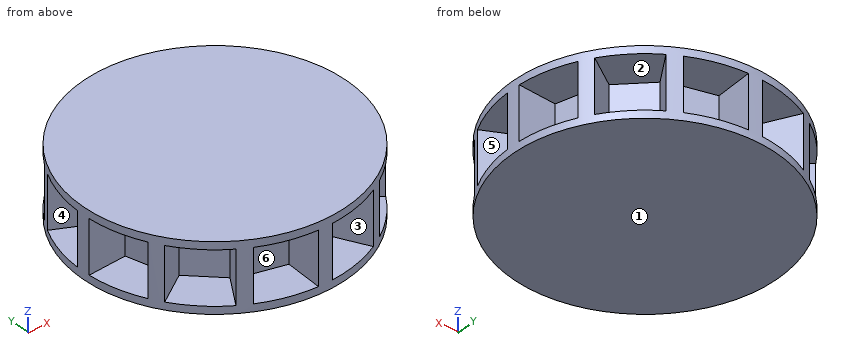
```python
from build123d import *

# Parameters (mm, degrees)
F0_R     = 35
F1_DEPTH = 18
F3_DEPTH = 16
F4_R     = 35
F5_DEPTH = 2


with BuildPart() as f1:
    # F0 (on Top) → F1 (new body)
    with BuildSketch(Plane.XY):
        Circle(F0_R)
    extrude(amount=F1_DEPTH)

    # F2 (on face) → F3 (cut)
    with BuildSketch(Plane(origin=(0, 0, 0), x_dir=(1, 0, 0), z_dir=(0, 0, -1))):
        with BuildLine():
            Line((11.3497624935, 22.2751631047), (15.8896674909, 31.1852283466))
            ThreePointArc((15.8896674909, 31.1852283466), (9.0586665786, 33.8074039201), (1.8317584685, 34.9520337164))
            Line((1.8317584685, 34.9520337164), (1.3083989061, 24.9657383689))
            Line((1.3083989061, 24.9657383689), (11.3497624935, 22.2751631047))
        make_face()
        with BuildLine():
            Line((20.9667641986, 13.6159758754), (29.3534698781, 19.0623662255))
            ThreePointArc((29.3534698781, 19.0623662255), (24.7487373415, 24.7487373415), (19.0623662255, 29.3534698781))
            Line((19.0623662255, 29.3534698781), (13.6159758754, 20.9667641986))
            Line((13.6159758754, 20.9667641986), (20.9667641986, 13.6159758754))
        make_face()
        with BuildLine():
            Line((24.9657383689, 1.3083989061), (34.9520337164, 1.8317584685))
            ThreePointArc((34.9520337164, 1.8317584685), (33.8074039201, 9.0586665786), (31.1852283466, 15.8896674909))
            Line((31.1852283466, 15.8896674909), (22.2751631047, 11.3497624935))
            Line((22.2751631047, 11.3497624935), (24.9657383689, 1.3083989061))
        make_face()
        with BuildLine():
            ThreePointArc((-31.1852283466, 15.8896674909), (-33.8074039201, 9.0586665786), (-34.9520337164, 1.8317584685))
            Line((-34.9520337164, 1.8317584685), (-24.9657383689, 1.3083989061))
            Line((-24.9657383689, 1.3083989061), (-22.2751631047, 11.3497624935))
            Line((-22.2751631047, 11.3497624935), (-31.1852283466, 15.8896674909))
        make_face()
        with BuildLine():
            ThreePointArc((-19.0623662255, 29.3534698781), (-24.7487373415, 24.7487373415), (-29.3534698781, 19.0623662255))
            Line((-29.3534698781, 19.0623662255), (-20.9667641986, 13.6159758754))
            Line((-20.9667641986, 13.6159758754), (-13.6159758754, 20.9667641986))
            Line((-13.6159758754, 20.9667641986), (-19.0623662255, 29.3534698781))
        make_face()
        with BuildLine():
            ThreePointArc((-1.8317584685, 34.9520337164), (-9.0586665786, 33.8074039201), (-15.8896674909, 31.1852283466))
            Line((-15.8896674909, 31.1852283466), (-11.3497624935, 22.2751631047))
            Line((-11.3497624935, 22.2751631047), (-1.3083989061, 24.9657383689))
            Line((-1.3083989061, 24.9657383689), (-1.8317584685, 34.9520337164))
        make_face()
        with BuildLine():
            ThreePointArc((-15.8896674909, -31.1852283466), (-9.0586665786, -33.8074039201), (-1.8317584685, -34.9520337164))
            Line((-1.8317584685, -34.9520337164), (-1.3083989061, -24.9657383689))
            Line((-1.3083989061, -24.9657383689), (-11.3497624935, -22.2751631047))
            Line((-11.3497624935, -22.2751631047), (-15.8896674909, -31.1852283466))
        make_face()
        with BuildLine():
            ThreePointArc((-29.3534698781, -19.0623662255), (-24.7487373415, -24.7487373415), (-19.0623662255, -29.3534698781))
            Line((-19.0623662255, -29.3534698781), (-13.6159758754, -20.9667641986))
            Line((-13.6159758754, -20.9667641986), (-20.9667641986, -13.6159758754))
            Line((-20.9667641986, -13.6159758754), (-29.3534698781, -19.0623662255))
        make_face()
        with BuildLine():
            ThreePointArc((-34.9520337164, -1.8317584685), (-33.8074039201, -9.0586665786), (-31.1852283466, -15.8896674909))
            Line((-31.1852283466, -15.8896674909), (-22.2751631047, -11.3497624935))
            Line((-22.2751631047, -11.3497624935), (-24.9657383689, -1.3083989061))
            Line((-24.9657383689, -1.3083989061), (-34.9520337164, -1.8317584685))
        make_face()
        with BuildLine():
            ThreePointArc((31.1852283466, -15.8896674909), (33.8074039201, -9.0586665786), (34.9520337164, -1.8317584685))
            Line((34.9520337164, -1.8317584685), (24.9657383689, -1.3083989061))
            Line((24.9657383689, -1.3083989061), (22.2751631047, -11.3497624935))
            Line((22.2751631047, -11.3497624935), (31.1852283466, -15.8896674909))
        make_face()
        with BuildLine():
            ThreePointArc((19.0623662255, -29.3534698781), (24.7487373415, -24.7487373415), (29.3534698781, -19.0623662255))
            Line((29.3534698781, -19.0623662255), (20.9667641986, -13.6159758754))
            Line((20.9667641986, -13.6159758754), (13.6159758754, -20.9667641986))
            Line((13.6159758754, -20.9667641986), (19.0623662255, -29.3534698781))
        make_face()
        with BuildLine():
            ThreePointArc((1.8317584685, -34.9520337164), (9.0586665786, -33.8074039201), (15.8896674909, -31.1852283466))
            Line((15.8896674909, -31.1852283466), (11.3497624935, -22.2751631047))
            Line((11.3497624935, -22.2751631047), (1.3083989061, -24.9657383689))
            Line((1.3083989061, -24.9657383689), (1.8317584685, -34.9520337164))
        make_face()
    extrude(amount=-F3_DEPTH, mode=Mode.SUBTRACT)

    # F4 (on face) → F5 (join)
    with BuildSketch(Plane(origin=(0, 0, 0), x_dir=(1, 0, 0), z_dir=(0, 0, -1))):
        Circle(F4_R)
    extrude(amount=-F5_DEPTH)


solid = f1.part
```
Read the model definition and answer for the solid it produces. Units are mm, in the model's axes. Face numbers are marked on the shaded views. A direction names the side the tool comes from. Coordinates: 2 decimals unless noted, no trailing zeros. Loops run counter-clockwise (first coordinate to the right, second up) from the corner with the lowest first, then second, coordinate; pieces in that order, holes last. Notation, with made-up numbers: (11.5, 65.25) - (29.5, 65.25) arc R28 ccw to (29.5, 101.25) - close; hole circle Ø5 at (29, 81). An arc over 180 degrees is marked (long way). Answer in a Markdown table with one row per item.
1. Which of the six approach directions +Z, -Z, +X, -X, +Y, -Y give full straight-line access (tool end or side, diameter ignored) to the marked faces 1, 2 and 3?
Conclusion:
| item | result |
|---|---|
| face 1 | -Z, +X, -X, +Y, -Y |
| face 2 | none |
| face 3 | -Y |
2. Find section D-D, the plane x = -6.5. Write down the section's boundary in (y, z), then the cut area to 3 significant figures.
Conclusion:
| item | result |
|---|---|
| outline | (-34.39, 0) - (34.39, 0) - (34.39, 2) - (23.57, 2) - (23.57, 16) - (34.39, 16) - (34.39, 18) - (-34.39, 18) - (-34.39, 16) - (-23.57, 16) - (-23.57, 2) - (-34.39, 2) - close |
| area | 935 mm² |
3. Determine the mould class of the marked faces 4, 5 and 6 for opening direction X: +X half, -X half, draft (parallel to the pull), parting line (faces both ways), or undercut.
Conclusion:
| item | result |
|---|---|
| face 4 | -X half |
| face 5 | +X half |
| face 6 | undercut |
4. Find section A-A, the plane x = -24. Write down the section's boundary in (y, z).
Conclusion:
| item | result |
|---|---|
| outline | (-25.48, 0) - (25.48, 0) - (25.48, 2) - (15.59, 2) - (15.59, 16) - (25.48, 16) - (25.48, 18) - (-25.48, 18) - (-25.48, 16) - (-15.59, 16) - (-15.59, 2) - (-25.48, 2) - close; hole (-12.23, 2) - (-4.91, 2) - (-4.91, 16) - (-12.23, 16) - close; hole (4.91, 2) - (12.23, 2) - (12.23, 16) - (4.91, 16) - close |
5. Given pin 1 (8 mm diameter, centred on y = 25.5, z = 13, fed in from +X); pin 2 (1.5 mm diameter, centred on x = -19.5, z = 15.5, fed in from -Y); pin 3 (1.5 mm diameter, centred on y = -16.5, z = 14.5, fed in from -X), each flat-ended and moving along its own axis, determine where each tip first touches the part or whether it passes through.
Conclusion:
| item | result |
|---|---|
| pin 1 | stops at x = 26.51 |
| pin 2 | stops at y = -29.55 |
| pin 3 | stops at x = -31.19 |
6. Find section B-B, the plane y = -5. Write down the section's boundary in (x, z).
Conclusion:
| item | result |
|---|---|
| outline | (-34.64, 0) - (34.64, 0) - (34.64, 2) - (23.98, 2) - (23.98, 16) - (34.64, 16) - (34.64, 18) - (-34.64, 18) - (-34.64, 16) - (-23.98, 16) - (-23.98, 2) - (-34.64, 2) - close |
7. Find section C-C, the plane y = -27. Write down the section's boundary in (x, z).
Conclusion:
| item | result |
|---|---|
| outline | (-22.27, 0) - (22.27, 0) - (22.27, 2) - (17.53, 2) - (17.53, 16) - (22.27, 16) - (22.27, 18) - (-22.27, 18) - (-22.27, 16) - (-17.53, 16) - (-17.53, 2) - (-22.27, 2) - close; hole (-13.76, 2) - (-1.42, 2) - (-1.42, 16) - (-13.76, 16) - close; hole (1.42, 2) - (13.76, 2) - (13.76, 16) - (1.42, 16) - close |
8. Straight lines are drawn through the part: line 1 (X direction, y = 15.5, z = 3.75); line 2 (Y direction, x = 25.5, z = 15.5); line 3 (Z direction, x = 18.5, y = -21). For each, find the intervals that lie inside material, in ascending order.
Conclusion:
| item | result |
|---|---|
| line 1 | x = -30.42 to -23.87, -19.08 to 19.08, 23.87 to 30.42 |
| line 2 | y = -16.56 to -12.99, -1.34 to 1.34, 12.99 to 16.56 |
| line 3 | z = 0 to 2, 16 to 18 |
